Build history of the part. All positions in model axes, mm. A direction names the side the tool comes from. Round coordinates to 2 decimals unless told otherwise and drop trailing zeros. Order: outer loops, then holes, each group sorted by start corner. A loop starts at its lowest first (then second) coordinate and runs counter-clockwise, first axis right, second up. Notation, with made-up numbers: M 88.5,26.25 L 93.5,26.25 A3 ccw 93.5,31.25 Z; hole C -38,-11.75 d9. An arc over 180 degrees is marked long. One line per item, written item: value. Start each with the question number.
Item 1: Band-saw the part on D-D, the plane x = 221. Write the cut outline in (y, z).
Item 2: Two-plate mould, pull along X, no slides. Class faces 4 (the flat face through (218.3, 8, 43)), 5 (the flat face through (231, 3, 45)), 6 (the cylindrical face through (234.26, 8.13, 40.85)): +X half, -X half, draft (parallel to the pull), parting line (faces both ways), or undercut.
Item 3: Band-saw the part on B-B, the plane y = 8.5. Write the cut outline in (x, z), then the cut area to 3 significant figures.
Item 4: Probe L1, parallel to Z at x = 229.7, y = 10.75; L2, parallel to Z at x = 227.75, y = 8.5; L3, parallel to Z at x = 229.7, y = 7.75. List the from-to ranges inside material, lowest first.
Item 5: Tool access for faces 1 (the flat face through (221, 12, 50)), 2 (the flat face through (231.614, 13.336, 45.311)), 3 (the flat face through (221, 10.5, 48)): list every direction of +Z, -Z, +X, -X, +Y, -Y with a clear straight run to the whole face (end or side of a thin tool).
Item 6: Band-saw the part on A-A, the plane x = 232.7. Write the cut outline in (y, z).
Item 7: Pin check, flat tips, straight feed: pin 1 (1.9 mm diameter, centred on x = 229.7, z = 54.5, fed in from +Y); pin 2 (2.5 mm diameter, centred on x = 222, y = 11.5, fed in from +Z); pin 3 (1.5 mm diameter, centred on x = 230.5, z = 55.5, fed in from -Y); pin 4 (2.5 mm diameter, centred on x = 221.5, y = 7.5, fed in from +Z). Stop position of each tip, or through.
```python
from build123d import *

# Parameters (mm, degrees)
CYLINDER181_R     = 2.1
CYLINDER181_DEPTH = 19
CYLINDER127_R     = 1.6
CYLINDER127_DEPTH = 40
CYLINDER124_R     = 1.6
CYLINDER124_DEPTH = 40
EXTRUDE067_DEPTH  = 5
EXTRUDE050_DEPTH  = 15
EXTRUDE049_DEPTH  = 21


with BuildPart() as cylinder181:
    # Cylinder181 → Cylinder181 (new body)
    with BuildSketch(Plane(origin=(15.3, 8.5, 48.5), x_dir=(0, 0, 1), z_dir=(-1, 0, 0))):
        Circle(CYLINDER181_R)
    extrude(amount=CYLINDER181_DEPTH)


with BuildPart() as cylinder127:
    # Cylinder127 → Cylinder127 (new body)
    with BuildSketch(Plane(origin=(5.3, 42, 40.5), x_dir=(0, 0, -1), z_dir=(0, -1, 0))):
        Circle(CYLINDER127_R)
    extrude(amount=CYLINDER127_DEPTH)


with BuildPart() as cylinder124:
    # Cylinder124 → Cylinder124 (new body)
    with BuildSketch(Plane(origin=(8.3, 42, 54.5), x_dir=(0, 0, -1), z_dir=(0, -1, 0))):
        Circle(CYLINDER124_R)
    extrude(amount=CYLINDER124_DEPTH)


with BuildPart() as extrude067:
    # Sketch055 → Extrude067 (new body)
    with BuildSketch(Plane.YZ):
        Polygon((3, 46), (10.5, 46), (10.5, 50), (13.646271, 50), (12.6, 35), (3, 35), align=None)
    extrude(amount=EXTRUDE067_DEPTH)


with BuildPart() as extrude067_1:
    # Extrude067 placement: moved
    add(extrude067.part.moved(Location((14.7, 0, 0))))


with BuildPart() as extrude050:
    # Sketch040 → Extrude050 (new body)
    with BuildSketch(Plane.XZ):
        Polygon((-8.16038, 62.64716), (-8.16038, 30.419451), (4.410427, 62.64716), align=None)
    extrude(amount=-EXTRUDE050_DEPTH)


with BuildPart() as extrude050_1:
    # Extrude050 placement: moved
    add(extrude050.part.moved(Location((0, 1.5, 0))))


with BuildPart() as cut276:
    # Sketch039 → Extrude049 (new body)
    with BuildSketch(Plane.YZ):
        Polygon((3, 62), (3, 35), (12.616711, 35), (14.5, 62), align=None)
    extrude(amount=EXTRUDE049_DEPTH)


with BuildPart() as cut276_1:
    # Extrude049 placement: moved
    add(cut276.part.moved(Location((-6.3, 0, 0))))

    # Cut273: cut Extrude050
    add(extrude050_1.part, mode=Mode.SUBTRACT)

    # Fusion115: union Extrude067
    add(extrude067_1.part)

    # Cut274: cut Cylinder124
    add(cylinder124.part, mode=Mode.SUBTRACT)

    # Cut275: cut Cylinder127
    add(cylinder127.part, mode=Mode.SUBTRACT)

    # Cut276: cut Cylinder181
    add(cylinder181.part, mode=Mode.SUBTRACT)


with BuildPart() as part_mirroring:
    # Part__Mirroring: instance of Cut276
    add(cut276_1.part.mirror(Plane(origin=(0, 8.75, 48.500027), x_dir=(0, -1, 0), z_dir=(1, 0, 0))))


with BuildPart() as part_mirroring_1:
    # Part__Mirroring placement: moved
    add(part_mirroring.part.moved(Location((238, 0, 0))))


solid = part_mirroring_1.part
```
Output:
1. outline: M 3,35 L 12.6,35 L 13.65,50 L 10.5,50 L 10.5,46 L 3,46 Z
2. face 4: -X half
2. face 5: draft
2. face 6: undercut
3. outline: M 218.3,35 L 244.3,35 L 244.3,35.19 L 239.93,46.4 L 223.3,46.4 L 223.3,46 L 218.3,46 Z; M 223.3,50.6 L 238.29,50.6 L 233.84,62 L 223.3,62 Z; hole C 229.7,54.5 d3.2; hole C 232.7,40.5 d3.2
3. area: 399 mm²
4. L1: z = 35 to 52.9, 56.1 to 62
4. L2: z = 35 to 46.4, 50.6 to 62
4. L3: z = 35 to 46.54, 50.46 to 52.9, 56.1 to 62
5. face 1: +Z, -X, +Y, -Y
5. face 2: -Z, +X, -X, +Y
5. face 3: +Z, -X, -Y
6. outline: M 3,35 L 12.62,35 L 12.89,38.9 L 3,38.9 Z; M 3,42.1 L 13.11,42.1 L 14.5,62 L 3,62 Z; hole C 8.5,48.5 d4.2
7. pin 1: passes through
7. pin 2: stops at z = 50
7. pin 3: stops at y = 3
7. pin 4: stops at z = 46
